Check sheet for the drawn part. Datum: minimum x, y, z corner. Units: mm. Coordinates: 2 decimals unless noted, no trailing zeros. Loops run counter-clockwise (first coordinate to the right, second up) from the corner with the lowest first, then second, coordinate; pieces in that order, holes last.
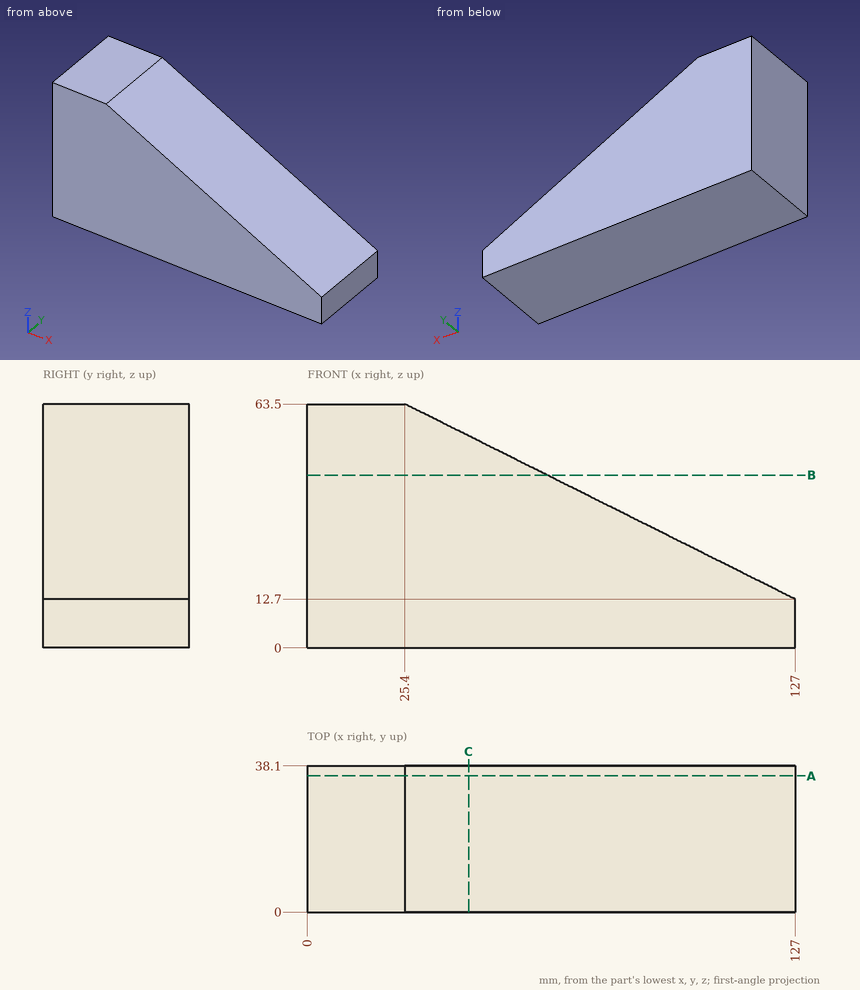
1) Depth check by flat-ended pin: pin 1 (5 mm diameter, centred on x = 71, y = 28, fed in from +Z); pin 2 (10 mm diameter, centred on x = 98, y = 7, fed in from +Z); pin 3 (10 mm diameter, centred on x = 57.5, y = 10.5, fed in from +Z). Enter the tip coordinate at first touch or a pass-through.
Answer sheet:
pin 1: stops at z = 41.95
pin 2: stops at z = 29.7
pin 3: stops at z = 49.95
2) Section check B-B on z = 45. Enter the section's corners in (x, y), plus the area to 3 significant figures.
Answer sheet:
outline: (0, 0) - (62.4, 0) - (62.4, 38.1) - (0, 38.1) - close
area: 2,380 mm2
3) Scan lines: line 1 (Z direction, x = 106.5, y = 31); line 2 (Z direction, x = 90.5, y = 29); line 3 (X direction, y = 20, z = 51). Record each from-to range of solid material in increasing order.
Answer sheet:
line 1: z = 0 to 22.95
line 2: z = 0 to 30.95
line 3: x = 0 to 50.4
4) Section check A-A on y = 35.5. Enter the section's corners in (x, z).
Answer sheet:
outline: (0, 0) - (127, 0) - (127, 12.7) - (25.4, 63.5) - (0, 63.5) - close
5) Section check C-C on x = 42. Enter the section's corners in (y, z).
Answer sheet:
outline: (0, 0) - (38.1, 0) - (38.1, 55.2) - (0, 55.2) - close
